Build history of the part. All positions in model axes, mm. A direction names the side the tool comes from. Give positions to 0.01 mm unless a question says otherwise; leave off trailing zeros. Loops run counter-clockwise (first coordinate to the right, second up) from the corner with the lowest first, then second, coordinate; pieces in that order, holes last.
1) Band-saw the part on D-D on x = 79.25. List the corners of the cut face in (y, z).
2) Band-saw the part on A-A on z = 3.5. List the corners of the cut face in (x, y).
3) Wall check: line 1 (X direction, y = 308.5, z = 5.75); line 2 (Y direction, x = 55, z = 3.5); line 3 (Y direction, x = 79.25, z = 4.25). Give the ranges that are in metal, low to high.
4) Band-saw the part on C-C on z = 6.75. List the corners of the cut face in (x, y).
5) Flat gauge pins, fed straight in: P1, Ø1, axis at y = 285, z = 6.5, coming from the +X side; P2, Ø5, axis at x = 65, y = 271, coming from the -Z side; P3, Ø1.4, axis at x = 37.5, z = 3, coming from the -Y side. Where does each tip first touch, or does it go through?
6) 3-axis set-ups, long thin cutter, end or side, ignore diameter. For faces 1 (the flat face through (35, 311, 3)), 2 (the flat face through (70.25, 323, 3)), 3 (the flat face through (55, 271.5, 4)), 4 (the flat face through (31.81, 322.05, 3.7)), 5 (the flat face through (50, 266, 3)): which of +Z, -Z, +X, -X, +Y, -Y reach the whole face in a straight line?
7) Band-saw the part on B-B on y = 308.5. List the corners of the cut face in (x, z), then the cut area to 3 significant figures.
8) Two-plate mould, pull along Z, no slides. Class faces 6 (the cylindrical face through (55.69, 264.67, 3.7)), 7 (the cylindrical face through (54.01, 270.74, 3.63)), 8 (the flat face through (78, 314, 0)): +Z half, -Z half, draft (parallel to the pull), parting line (faces both ways), or undercut.
```python
from build123d import *

# Parameters (mm, degrees)
SKETCH_1_R        = 1.5
EXTRUDE_1_DEPTH   = 6
EXTRUDE_1_2_DEPTH = 6
SKETCH_1_W        = 10
SKETCH_1_H        = 7
EXTRUDE_1_3_DEPTH = 6
SKETCH_2_R        = 1.5
EXTRUDE_2_DEPTH   = 1.5
SKETCH_3_R        = 1
EXTRUDE_3_DEPTH   = 1.5


with BuildPart() as part:
    # Sketch 1 → Extrude 1 (new body)
    with BuildSketch(Plane.XY):
        Polygon((39.75, 326), (39.75, 321), (35, 321), (35, 301), (27.75, 301), (27.75, 317.992640687), (35.757359313, 326), align=None)
        with Locations((30.75, 308.5)):
            Circle(SKETCH_1_R, mode=Mode.SUBTRACT)
    extrude(amount=EXTRUDE_1_DEPTH)



with BuildPart() as body_2:
    # Sketch 1 → Extrude 1 2 (new body)
    with BuildSketch(Plane.XY):
        Polygon((82.25, 301), (75, 301), (75, 321), (70.25, 321), (70.25, 326), (74.242640687, 326), (82.25, 317.992640687), align=None)
        with Locations((79.25, 308.5)):
            Circle(SKETCH_1_R, mode=Mode.SUBTRACT)
    extrude(amount=EXTRUDE_1_2_DEPTH)


with BuildPart() as body_3:
    # Sketch 1 → Extrude 1 3 (new body)
    with BuildSketch(Plane.XY):
        with Locations((55, 266.5)):
            Rectangle(SKETCH_1_W, SKETCH_1_H)
        with Locations((55, 266)):
            Circle(SKETCH_1_R, mode=Mode.SUBTRACT)
    extrude(amount=EXTRUDE_1_3_DEPTH)


with BuildPart() as part_1:
    add(part.part)

    add(body_2.part)  # Extrude 2 merges body 2

    add(body_3.part)  # Extrude 2 merges body 3
    # Sketch 2 → Extrude 2 (add)
    with BuildSketch(Plane.XY.offset(6)):
        Polygon((82.25, 301), (82.25, 317.992640687), (74.242640687, 326), (70.25, 326), (39.75, 326), (35.757359313, 326), (27.75, 317.992640687), (27.75, 301), (50, 263), (60, 263), align=None)
        with Locations((55, 266)):
            Circle(SKETCH_2_R, mode=Mode.SUBTRACT)
        with Locations((79.25, 308.5)):
            Circle(SKETCH_2_R, mode=Mode.SUBTRACT)
        with Locations((30.75, 308.5)):
            Circle(SKETCH_2_R, mode=Mode.SUBTRACT)
    extrude(amount=EXTRUDE_2_DEPTH)

    # Sketch 3 → Extrude 3 (add)
    with BuildSketch(Plane(origin=(0, 270, 0), x_dir=(1, 0, 0), z_dir=(0, 1, 0))):
        with Locations(Location((55, -3.5, 0), (0, 0, 90))):
            Circle(SKETCH_3_R)
    extrude(amount=EXTRUDE_3_DEPTH)


solid = part_1.part
```
Findings below:
1. outline: (295.88, 6) - (301, 6) - (301, 0) - (307, 0) - (307, 7.5) - (295.88, 7.5) - close; (310, 0) - (320.99, 0) - (320.99, 7.5) - (310, 7.5) - close
2. outline: (27.75, 301) - (35, 301) - (35, 321) - (39.75, 321) - (39.75, 326) - (35.76, 326) - (27.75, 317.99) - close; (50, 263) - (60, 263) - (60, 270) - (56, 270) - (56, 271.5) - (54, 271.5) - (54, 270) - (50, 270) - close; (70.25, 321) - (75, 321) - (75, 301) - (82.25, 301) - (82.25, 317.99) - (74.24, 326) - (70.25, 326) - close; hole circle Ø3 at (30.75, 308.5); hole circle Ø3 at (55, 266); hole circle Ø3 at (79.25, 308.5)
3. line 1: x = 27.75 to 29.25, 32.25 to 35, 75 to 77.75, 80.75 to 82.25
3. line 2: y = 263 to 264.5, 267.5 to 271.5
3. line 3: y = 301 to 307, 310 to 320.99
4. outline: (27.75, 301) - (50, 263) - (60, 263) - (82.25, 301) - (82.25, 317.99) - (74.24, 326) - (35.76, 326) - (27.75, 317.99) - close; hole circle Ø3 at (30.75, 308.5); hole circle Ø3 at (55, 266); hole circle Ø3 at (79.25, 308.5)
5. P1: stops at x = 73.17
5. P2: stops at z = 6
5. P3: stops at y = 321
6. face 1: -Z, -Y
6. face 2: -Z, +Y, -Y
6. face 3: -Z, +X, -X, +Y
6. face 4: +Z, -Z, -X, +Y
6. face 5: -Z, -X, +Y, -Y
7. outline: (27.75, 0) - (29.25, 0) - (29.25, 7.5) - (27.75, 7.5) - close; (32.25, 0) - (35, 0) - (35, 6) - (75, 6) - (75, 0) - (77.75, 0) - (77.75, 7.5) - (32.25, 7.5) - close; (80.75, 0) - (82.25, 0) - (82.25, 7.5) - (80.75, 7.5) - close
7. area: 124 mm2
8. face 6: draft
8. face 7: undercut
8. face 8: -Z half
